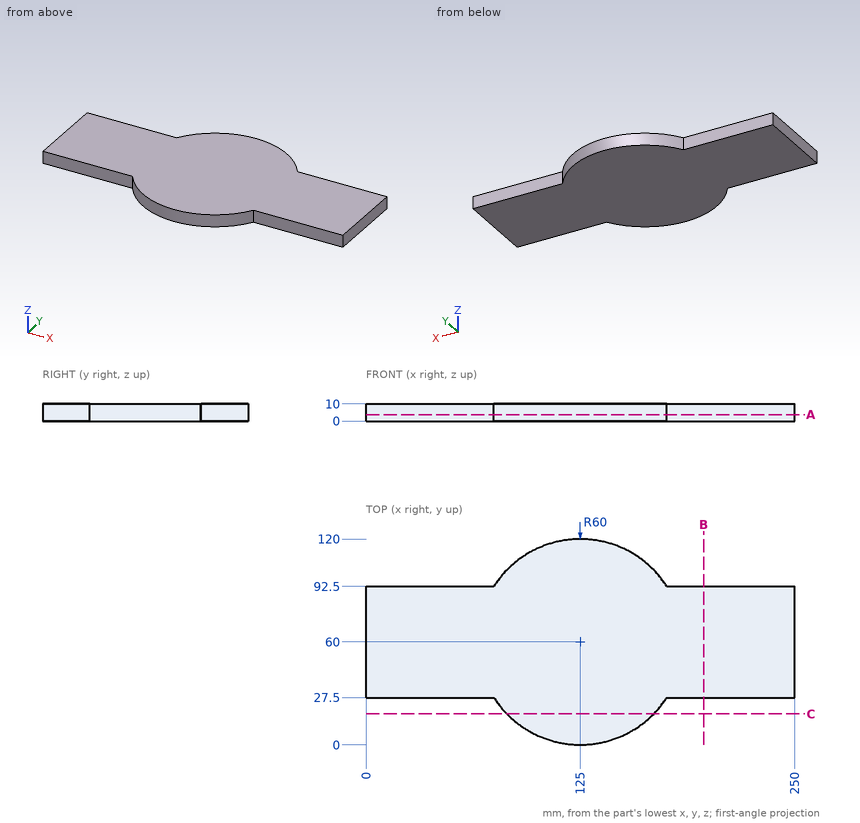
Source: three-view drawing plus pictorial views. Frame: mm from the lowest corner of the part. Round coordinates to 2 decimals unless told otherwise and drop trailing zeros. Write each loop counter-clockwise with the first axis right and the second up, starting at its lowest first coordinate (ties: lowest second). Pieces come first, ordered by that corner, then holes. Notation, with made-up numbers: M 85.5,1 L 144.5,1 A29 cw 144.5,26 Z; hole C 32.5,-26.75 d7. An arc over 180 degrees is marked long. One line per item, written item: value. Start each with the question number.
Item 1: Ray query, L1, parallel to Y at x = 51, z = 4.5; L2, parallel to X at y = 12, z = 9; L3, parallel to Y at x = 120, z = 7. Return the intervals inside material, ascending. Write a range as from..to.
Item 2: Pin query (flat end, axial travel): pin 1 (5 mm diameter, centred on x = 216.5, z = 5.5, fed in from -Y); pin 2 (5 mm diameter, centred on x = 219, z = 6, fed in from +Y); pin 3 (1 mm diameter, centred on x = 111.5, z = 8.5, fed in from +Y). Return the tip coordinate at first contact, or that it passes through.
Item 3: Section query C-C (y = 18). Return the cut outline in (x, z), plus the area to 3 significant figures.
Item 4: Section query B-B (x = 197). Return the cut outline in (y, z).
Item 5: Section query A-A (z = 3.75). Return the cut outline in (x, y).
Result set:
1. L1: y = 27.5..92.5
1. L2: x = 89..161
1. L3: y = 0.21..119.79
2. pin 1: stops at y = 27.5
2. pin 2: stops at y = 92.5
2. pin 3: stops at y = 118.57
3. outline: M 82.15,0 L 167.85,0 L 167.85,10 L 82.15,10 Z
3. area: 857 mm²
4. outline: M 27.5,0 L 92.5,0 L 92.5,10 L 27.5,10 Z
5. outline: M 0,27.5 L 74.56,27.5 A60 ccw 175.44,27.5 L 250,27.5 L 250,92.5 L 175.44,92.5 A60 ccw 74.56,92.5 L 0,92.5 Z
